For this review, take the finished solid that the model builds, in its own axes (mm). Give positions to 0.01 mm unless a question says otherwise; leave off trailing zeros. Order: outer loops, then holes, each group sorted by start corner. A loop starts at its lowest first (then second) coordinate and runs counter-clockwise, first axis right, second up. Notation, with made-up numbers: (31, 70) -> (40, 70) arc R9 ccw to (40, 87) -> close; hole circle Ø11 at (38.25, 30). An arc over 180 degrees is marked (long way). Return JSON: item names as keys, results as strings. Group by question number.
1) Insertion check: P1, Ø6, axis at x = 54.5, z = -17.5, coming from the -Y side; P2, Ø5, axis at x = 63.5, z = -38.1, coming from the +Y side. Each pin has a flat end and moves straight along its axis. Give the tip position at first contact, or say it passes through.
2) The part is to be moulded in two halves that separate along Z. For faces 1 (the face through (0, 2, -25)), 2 (the face through (65.73, 0.95, -25.89)), 3 (the face through (63, 2, -50.8)), say which applies: released by +Z, released by -Z, zero draft, split by the parting line, or undercut.
3) Add section B-B (z = -25.4). Give the boundary of the cut face in (x, y) (3 decimals).
4) To check wall thickness, follow line 1 along X through (y, z) = (0.45, -25.4) (3 decimals); line 2 along Z through (x, y) = (63.5, 0.5); line 3 along Z through (x, y) = (63, 2.15). State the ranges of each line that lie inside material, in increasing order.
5) Add section A-A (x = 63.5). Give the boundary of the cut face in (y, z) (3 decimals), then the cut area to 3 significant figures.
6) Add section D-D (z = -38.1). Give the boundary of the cut face in (x, y) (3 decimals).
7) Add section C-C (x = 114.3). Give the boundary of the cut face in (y, z) (3 decimals).
from build123d import *

# Parameters (mm, degrees)
SKETCH1_W                                     = 127
SKETCH1_H                                     = 50.8
BOSS_EXTRUDE1_DEPTH                           = 3.175
SKETCH2_R                                     = 3.175
CUT_EXTRUDE1_DEPTH                            = 6.35
CSK_FOR_8_FLAT_HEAD_MACHINE_SCREW1_AT_2_COUNT = 2
CSK_FOR_8_FLAT_HEAD_MACHINE_SCREW1_AT_2_PITCH = 12.7
CSK_FOR_8_FLAT_HEAD_MACHINE_SCREW1_AT_3_COUNT = 2
CSK_FOR_8_FLAT_HEAD_MACHINE_SCREW1_AT_3_PITCH = 25.4


with BuildPart() as part:
    # Sketch1 → Boss-Extrude1 (new body)
    with BuildSketch(Plane(origin=(0, 0, 0), x_dir=(1, 0, 0), z_dir=(0, 1, 0))):
        with Locations((63.5, 25.4)):
            Rectangle(SKETCH1_W, SKETCH1_H)
    extrude(amount=BOSS_EXTRUDE1_DEPTH)

    # Sketch2 → Cut-Extrude1 (cut)
    with BuildSketch(Plane(origin=(0, 3.175, 0), x_dir=(1, 0, 0), z_dir=(0, 1, 0))):
        with Locations(Location((12.7, 25.4, 0), (0, 0, 270))):
            Circle(SKETCH2_R)
        with Locations(Location((114.3, 25.4, 0), (0, 0, 270))):
            Circle(SKETCH2_R)
    extrude(amount=-CUT_EXTRUDE1_DEPTH, mode=Mode.SUBTRACT)

    # Sketch4 → CSK for #8 Flat Head Machine Screw1 (revolve, cut)
    with BuildSketch(Plane(origin=(63.5, 3.175, -12.7), x_dir=(0, 0, 1), z_dir=(1, 0, 0))):
        Polygon((0, 0), (0, 3.175), (2.15265, 3.175), (2.15265, 2.3740728), (4.2164, 0), align=None)
    csk_for_8_flat_head_machine_screw1 = revolve(axis=Axis((63.5, 9.525, -12.7), (0, -1, 0)), mode=Mode.SUBTRACT)

    # CSK for #8 Flat Head Machine Screw1 at 2: CSK for #8 Flat Head Machine Screw1 ×2
    with Locations(*[(0, 0, -i * CSK_FOR_8_FLAT_HEAD_MACHINE_SCREW1_AT_2_PITCH) for i in range(1, CSK_FOR_8_FLAT_HEAD_MACHINE_SCREW1_AT_2_COUNT)]):
        add(csk_for_8_flat_head_machine_screw1, mode=Mode.SUBTRACT)

    # CSK for #8 Flat Head Machine Screw1 at 3: CSK for #8 Flat Head Machine Screw1 ×2
    with Locations(*[(0, 0, -i * CSK_FOR_8_FLAT_HEAD_MACHINE_SCREW1_AT_3_PITCH) for i in range(1, CSK_FOR_8_FLAT_HEAD_MACHINE_SCREW1_AT_3_COUNT)]):
        add(csk_for_8_flat_head_machine_screw1, mode=Mode.SUBTRACT)


solid = part.part
Evaluation:
{
 "1": {"P1": "y = 0", "P2": "y = 1.2"},
 "2": {"face 1": "zero draft", "face 2": "undercut", "face 3": "released by -Z"},
 "3": {"outline": "(0, 0) -> (9.525, 0) -> (9.525, 3.175) -> (0, 3.175) -> close; (15.875, 0) -> (61.347, 0) -> (61.347, 0.801) -> (59.284, 3.175) -> (15.875, 3.175) -> close; (65.653, 0) -> (111.125, 0) -> (111.125, 3.175) -> (67.716, 3.175) -> (65.653, 0.801) -> close; (117.475, 0) -> (127, 0) -> (127, 3.175) -> (117.475, 3.175) -> close"},
 "4": {"line 1": "0 to 9.525, 15.875 to 61.347, 65.653 to 111.125, 117.475 to 127", "line 2": "-50.8 to -40.25, -35.95 to -27.55, -23.25 to -14.85, -10.55 to 0", "line 3": "-50.8 to -41.39, -34.81 to -28.69, -22.11 to -15.99, -9.41 to 0"},
 "5": {"outline": "(0, -50.8) -> (3.175, -50.8) -> (3.175, -42.316) -> (0.801, -40.253) -> (0, -40.253) -> close; (0, -35.947) -> (0.801, -35.947) -> (3.175, -33.884) -> (3.175, -29.616) -> (0.801, -27.553) -> (0, -27.553) -> close; (0, -23.247) -> (0.801, -23.247) -> (3.175, -21.184) -> (3.175, -16.916) -> (0.801, -14.853) -> (0, -14.853) -> close; (0, -10.547) -> (0.801, -10.547) -> (3.175, -8.484) -> (3.175, 0) -> (0, 0) -> close", "area": "106 mm^2"},
 "6": {"outline": "(0, 0) -> (61.347, 0) -> (61.347, 0.801) -> (59.284, 3.175) -> (0, 3.175) -> close; (65.653, 0) -> (127, 0) -> (127, 3.175) -> (67.716, 3.175) -> (65.653, 0.801) -> close"},
 "7": {"outline": "(0, -50.8) -> (3.175, -50.8) -> (3.175, -28.575) -> (0, -28.575) -> close; (0, -22.225) -> (3.175, -22.225) -> (3.175, 0) -> (0, 0) -> close"}
}
